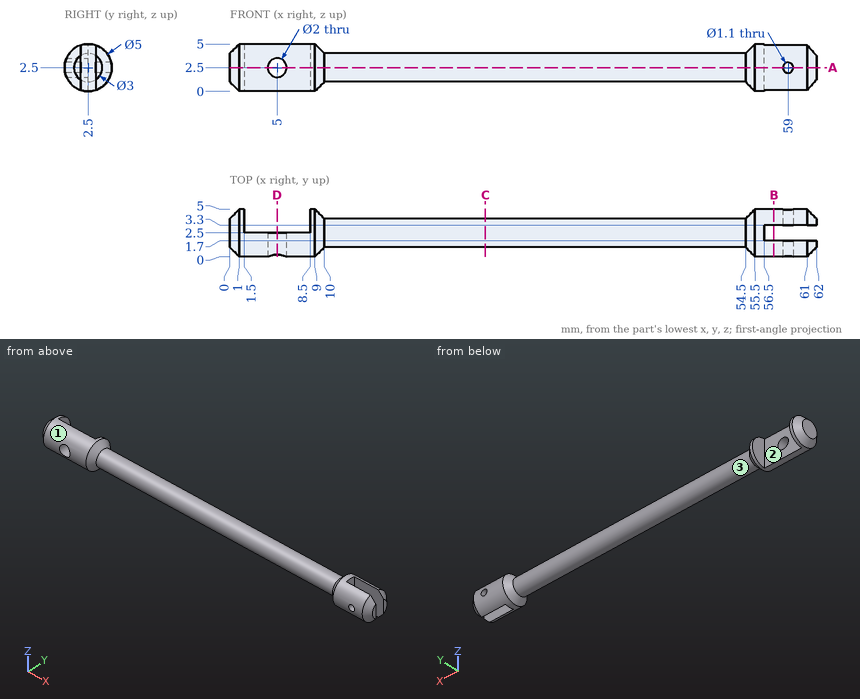
Answer from the drawing. Dimensions are ordinates in mm from the lowest x, y and z of the part. Round coordinates to 2 decimals unless told otherwise and drop trailing zeros. Write each loop counter-clockwise with the first axis right and the second up, starting at its lowest first coordinate (ties: lowest second). Pieces come first, ordered by that corner, then holes. Notation, with made-up numbers: M 33.25,53 L 86.25,53 A8 cw 86.25,57 Z; hole C -1,62.25 d8. An arc over 180 degrees is marked long. Write each question's results on one line, items separated by ' | '. Start each with the question number.
Item 1: A cutting plane is placed at A-A on z = 2.5. State how many separate pieces and enclosed holes the cut face has, and give its area (3 significant figures).
Item 2: A cutting plane is placed at B-B on x = 57.5. Write down the section's boundary in (y, z), and give its area (3 significant figures).
Item 3: Flat-ended cylindrical pins translate along their axes: pin 1 Ø3 at (x, y) = (50, 3.5) entering from -Z; pin 2 Ø0.8 at (y, z) = (2.5, 3.5) entering from +X; pin 3 Ø3 at (x, y) = (30.5, 1) entering from +Z. Find the tip coordinate at first contact, or state that the pin passes through.
Item 4: For a pull along X with two mould halves and no side action, classify the marked faces 1, 2 and 3 as pulls with the +X half, pulls with the -X half, needs draft (parallel to the pull), parting line crosses it, or undercut.
Item 5: A cutting plane is placed at C-C on x = 27. Write down the section's boundary in (y, z).
Item 6: A cutting plane is placed at D-D on x = 5. Write down the section's boundary in (y, z), and give its area (3 significant figures).
Item 7: Straight lines are drawn through the part: L1, parallel to X at y = 2.95, z = 0.6; L2, parallel to X at y = 4.35, z = 1.05; L3, parallel to Z at x = 59, y = 4.5. For each, find the intervals that lie inside material, in ascending order. Write a range as [from, to].
Check sheet entries:
1) separate pieces: 4 | enclosed holes: 0 | area: 182 mm²
2) outline: M 1.7,0.13 L 1.7,4.87 A2.5 ccw Z; M 3.3,0.13 A2.5 ccw 3.3,4.87 Z | area: 11.8 mm²
3) pin 1: z = 1 | pin 2: x = 56.5 | pin 3: z = 4
4) face 1: needs draft | face 2: undercut | face 3: undercut
5) outline: C 2.5,2.5 d3
6) outline: M 0.21,1.5 A2.5 ccw 2.5,0 L 2.5,1.5 Z; M 0.21,3.5 L 2.5,3.5 L 2.5,5 A2.5 ccw Z | area: 4.95 mm²
7) L1: [0.45, 1.5], [8.5, 9.55], [54.95, 56.5] | L2: [0.85, 1.5], [8.5, 9.15], [55.35, 61.15] | L3: [1, 1.95], [3.05, 4]
